Part model, mm, in its own coordinate system. A direction names the side the tool comes from. Round coordinates to 2 decimals unless told otherwise and drop trailing zeros. Order: outer loops, then holes, each group sorted by start corner. A loop starts at its lowest first (then second) coordinate and runs counter-clockwise, first axis right, second up. Notation, with made-up numbers: (48.5, -28.75) - (86.5, -28.75) arc R23 ccw to (86.5, 8.25) - close; hole circle Ø10 at (51, 39). An arc over 180 degrees is marked (long way). Return JSON: item names as keys, results as strings. Group by question number.
Item 1: Saw through at C-C on y = 0.4. List the corners of the cut face in (x, z), and give its area (3 significant figures).
Item 2: Drop flat-ended pins along their axis: pin 1 (1.5 mm diameter, centred on x = -3.5, y = 0.5, fed in from -Z); pin 2 (2 mm diameter, centred on y = 2.5, z = 3.5, fed in from +X); pin 3 (1.6 mm diameter, centred on y = 2, z = -3.5, fed in from +X). Give the stop position or say it passes through.
Item 3: Saw through at B-B on z = 0. List the corners of the cut face in (x, y).
Item 4: Saw through at A-A on x = 0. List the corners of the cut face in (y, z), and give its area (3 significant figures).
Item 5: Tool access for faces 4 (the face through (1.64, 1.97, 1.61)), 5 (the face through (2, 0, 0)): list every direction of +Z, -Z, +X, -X, +Y, -Y with a clear straight run to the whole face (end or side of a thin tool).
Item 6: Probe probe 1 along X at (y, z) = (2.95, 0); probe 2 along Z at (x, y) = (1.75, 0.45); probe 3 along X at (y, z) = (0.75, -2). List the from-to ranges inside material, lowest first.
Item 7: Two-plate mould, pull along X, no slides. Class faces 1 (the face through (0.35, 2, 3)), 2 (the face through (-4.88, 1.97, -1.08)), 3 (the face through (2, 4, 0)): released by +X, released by -X, zero draft, split by the parting line, or undercut.
Item 8: Saw through at D-D on x = 1. List the corners of the cut face in (y, z).
```python
from build123d import *

# Parameters (mm, degrees)
SKETCH_1_R      = 5
SKETCH_1_R_2    = 1.6
EXTRUDE_1_DEPTH = 4


with BuildPart() as part:
    # 草图1 → 凸台-拉伸1 (new body)
    with BuildSketch(Plane(origin=(0, 0, 0), x_dir=(1, 0, 0), z_dir=(0, 1, 0))):
        with Locations(Location((0, 0, 0), (0, 0, 270))):
            Circle(SKETCH_1_R)
        with Locations(Location((0, 0, 0), (0, 0, 270))):
            Circle(SKETCH_1_R_2, mode=Mode.SUBTRACT)
        with BuildLine():
            Line((2.273213584, 0.35), (4.285732143, 0.35))
            ThreePointArc((4.285732143, 0.35), (3.040559159, 3.040559159), (0.35, 4.285732143))
            Line((0.35, 4.285732143), (0.35, 2.273213584))
            ThreePointArc((0.35, 2.273213584), (1.626345597, 1.626345597), (2.273213584, 0.35))
        make_face(mode=Mode.SUBTRACT)
        with BuildLine():
            Line((4.285732143, -0.35), (2.273213584, -0.35))
            ThreePointArc((2.273213584, -0.35), (1.626345597, -1.626345597), (0.35, -2.273213584))
            Line((0.35, -2.273213584), (0.35, -4.285732143))
            ThreePointArc((0.35, -4.285732143), (3.040559159, -3.040559159), (4.285732143, -0.35))
        make_face(mode=Mode.SUBTRACT)
        with BuildLine():
            Line((-0.35, -4.285732143), (-0.35, -2.273213584))
            ThreePointArc((-0.35, -2.273213584), (-1.626345597, -1.626345597), (-2.273213584, -0.35))
            Line((-2.273213584, -0.35), (-4.285732143, -0.35))
            ThreePointArc((-4.285732143, -0.35), (-3.040559159, -3.040559159), (-0.35, -4.285732143))
        make_face(mode=Mode.SUBTRACT)
        with BuildLine():
            Line((-4.285732143, 0.35), (-2.273213584, 0.35))
            ThreePointArc((-2.273213584, 0.35), (-1.626345597, 1.626345597), (-0.35, 2.273213584))
            Line((-0.35, 2.273213584), (-0.35, 4.285732143))
            ThreePointArc((-0.35, 4.285732143), (-3.040559159, 3.040559159), (-4.285732143, 0.35))
        make_face(mode=Mode.SUBTRACT)
    extrude(amount=EXTRUDE_1_DEPTH)


solid = part.part
```
Filled in:
{
 "1": {"outline": "circle Ø10 at (0, 0); hole (-4.29, -0.35) arc R4.3 ccw to (-0.35, -4.29) - (-0.35, -2.27) arc R2.3 cw to (-2.27, -0.35) - close; hole (-4.29, 0.35) - (-2.27, 0.35) arc R2.3 cw to (-0.35, 2.27) - (-0.35, 4.29) arc R4.3 ccw to start; hole circle Ø3.2 at (0, 0); hole (0.35, -4.29) arc R4.3 ccw to (4.29, -0.35) - (2.27, -0.35) arc R2.3 cw to (0.35, -2.27) - close; hole (0.35, 2.27) arc R2.3 cw to (2.27, 0.35) - (4.29, 0.35) arc R4.3 ccw to (0.35, 4.29) - close", "area": "34.6 mm^2"},
 "2": {"pin 1": "stops at z = -4.18", "pin 2": "stops at x = 4.33", "pin 3": "stops at x = 4.21"},
 "3": {"outline": "(-5, 0) - (-1.6, 0) - (-1.6, 4) - (-5, 4) - close; (1.6, 0) - (5, 0) - (5, 4) - (1.6, 4) - close"},
 "4": {"outline": "(0, -5) - (4, -5) - (4, -1.6) - (0, -1.6) - close; (0, 1.6) - (4, 1.6) - (4, 5) - (0, 5) - close", "area": "27.2 mm^2"},
 "5": {"face 4": "+Y, -Y", "face 5": "+Z, -Z, +X, -X, -Y"},
 "6": {"probe 1": "x = -5 to -1.6, 1.6 to 5", "probe 2": "z = -4.68 to -3.93, -1.49 to 1.49, 3.93 to 4.68", "probe 3": "x = -4.58 to -3.81, -1.14 to 1.14, 3.81 to 4.58"},
 "7": {"face 1": "undercut", "face 2": "split by the parting line", "face 3": "zero draft"},
 "8": {"outline": "(0, -4.9) - (4, -4.9) - (4, -4.18) - (0, -4.18) - close; (0, -2.07) - (4, -2.07) - (4, -1.25) - (0, -1.25) - close; (0, 1.25) - (4, 1.25) - (4, 2.07) - (0, 2.07) - close; (0, 4.18) - (4, 4.18) - (4, 4.9) - (0, 4.9) - close"}
}
